```python
from build123d import *

# Parameters (mm, degrees)
F0_W     = 30
F0_H     = 14
F0_R     = 8
F1_DEPTH = 1.5


# Not quite as in the source:
# - a feature names something its author has since deleted; it is built from what else it names


with BuildPart() as f1:
    # F0 (on Front) → F1 (new body, symmetric)
    with BuildSketch(Plane.XZ):
        Polygon((-30, -2.9994321861), (0, -2.9994321861), (0, 0), (30, 0), (30, -2.9994321861), (57, -2.9994321861), (57, 114.0005678139), (30, 114.0005678139), (30, 117.0005678139), (0, 117.0005678139), (0, 114.0005678139), (-30, 114.0005678139), (-30, 117.0005678139), (-60, 117.0005678139), (-60, 0), (-30, 0), align=None)
        with Locations((0, 14.8116284981)):
            Rectangle(F0_W, F0_H, mode=Mode.SUBTRACT)
        with Locations((-13, 75.2281695604)):
            Circle(F0_R, mode=Mode.SUBTRACT)
        with Locations((13, 75.2218647463)):
            Circle(F0_R, mode=Mode.SUBTRACT)
    extrude(amount=F1_DEPTH, both=True)


solid = f1.part
```
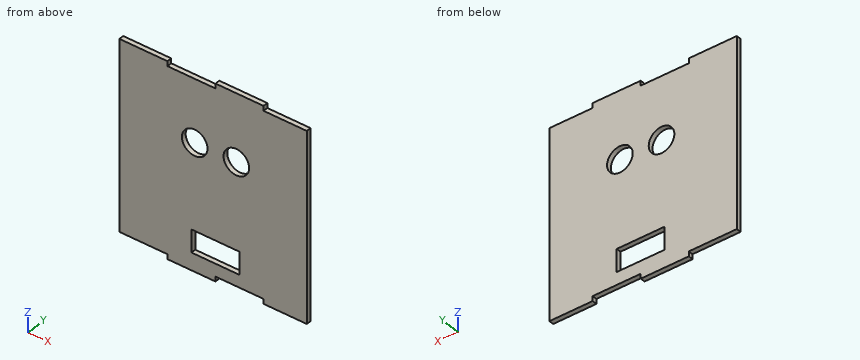
The listing builds one solid part. Answer for the finished solid, in the listing's coordinates (mm). Round coordinates to 2 decimals unless told otherwise and drop trailing zeros. Write each loop counter-clockwise with the first axis right and the second up, starting at its lowest first coordinate (ties: lowest second). Pieces come first, ordered by that corner, then holes. Notation, with made-up numbers: (-7, -11.75) -> (29, -11.75) arc R22 cw to (29, 22.25) -> close; hole circle Ø9 at (22, 75). An arc over 180 degrees is marked (long way). Answer as a JSON object with one key per item and string values. Group by question number.
Q1. Section B-B (z = 12.5) is taken. Write down the section's boundary in (x, y).
Q2. Section D-D (y = 0.35) is taken. Write down the section's boundary in (x, z).
Q3. Section C-C (z = 78) is taken. Write down the section's boundary in (x, y), plus the area to 3 significant figures.
Q4. Each of these flat-tipped pins is pushed along its axis until it touches: pin 1 Ø1.5 at (y, z) = (-0.5, -2) entering from -X; pin 2 Ø1.5 at (x, y) = (-15, 0) entering from +Z; pin 3 Ø1.5 at (x, y) = (16.5, 1) entering from -Z. Where does it stop, or does it pass through?
Q5. Section A-A (x = 13) is taken. Write down the section's boundary in (y, z).
Q6. Straight lines are drawn through the part: line 1 along Z through (x, y) = (13, -0.3); line 2 along Z through (x, y) = (-13, 0.15); line 3 along Z through (x, y) = (-2, -0.35). For each, find the intervals that lie inside material, in ascending order.
Check values:
{
 "1": {"outline": "(-60, -1.5) -> (-15, -1.5) -> (-15, 1.5) -> (-60, 1.5) -> close; (15, -1.5) -> (57, -1.5) -> (57, 1.5) -> (15, 1.5) -> close"},
 "2": {"outline": "(-60, 0) -> (-30, 0) -> (-30, -3) -> (0, -3) -> (0, 0) -> (30, 0) -> (30, -3) -> (57, -3) -> (57, 114) -> (30, 114) -> (30, 117) -> (0, 117) -> (0, 114) -> (-30, 114) -> (-30, 117) -> (-60, 117) -> close; hole circle Ø16 at (-13, 75.23); hole (-15, 7.81) -> (15, 7.81) -> (15, 21.81) -> (-15, 21.81) -> close; hole circle Ø16 at (13, 75.22)"},
 "3": {"outline": "(-60, -1.5) -> (-20.5, -1.5) -> (-20.5, 1.5) -> (-60, 1.5) -> close; (-5.5, -1.5) -> (5.5, -1.5) -> (5.5, 1.5) -> (-5.5, 1.5) -> close; (20.5, -1.5) -> (57, -1.5) -> (57, 1.5) -> (20.5, 1.5) -> close", "area": "261 mm^2"},
 "4": {"pin 1": "x = -30", "pin 2": "z = 114", "pin 3": "z = 0"},
 "5": {"outline": "(-1.5, 0) -> (1.5, 0) -> (1.5, 7.81) -> (-1.5, 7.81) -> close; (-1.5, 21.81) -> (1.5, 21.81) -> (1.5, 67.22) -> (-1.5, 67.22) -> close; (-1.5, 83.22) -> (1.5, 83.22) -> (1.5, 117) -> (-1.5, 117) -> close"},
 "6": {"line 1": "0 to 7.81, 21.81 to 67.22, 83.22 to 117", "line 2": "-3 to 7.81, 21.81 to 67.23, 83.23 to 114", "line 3": "-3 to 7.81, 21.81 to 114"}
}
